Autodesk Inventor part; units mm, degrees
ref_plane "YZ Plane" through (0, 0, 0) normal (1, 0, 0) x (0, 1, 0)
ref_plane "XZ Plane" through (0, 0, 0) normal (0, 1, 0) x (-1, 0, 0)
ref_plane "XY Plane" through (0, 0, 0) normal (0, 0, 1) x (1, 0, 0)
sketch "スケッチ1" plane through (0, 0, 0) normal (0, 1, 0) x (-1, 0, 0)
  arc A0 (-16.7033, 11) -> (16.7033, 11) centre (0, 0) ccw
  line L0 (16.7033, 11) -> (-16.7033, 11)
  point P0 (0, 11)
  dimension "d0" = 40
  dimension "d1" = 11
extrude "押し出し1" add sketch "スケッチ1" along normal blind 6
sketch "スケッチ3" plane through (0, 6, 0) normal (0, 1, 0) x (1, 0, 0)
  arc A0 (2.6833, -3.1) -> (-2.6833, -3.1) centre (0, 0) ccw
  line L0 (-2.6833, -3.1) -> (2.6833, -3.1)
  point P0 (0, -3.1)
  dimension "d12" = 8.2
  dimension "d13" = 3.1
extrude "押し出し2" cut sketch "スケッチ3" against normal blind 6
sketch "スケッチ4" plane through (0, 6, 0) normal (0, 1, 0) x (1, 0, 0)
  circle A0 centre (0, 0) radius 15.5 construction
  line L0 (0, 0) -> (-19.4826, 11.2483) construction
  line L1 (0, 0) -> (29.419, 16.9851) construction
  line L2 (0, 0) -> (0, 25.14) construction
  point P0 (0, 15.5)
  point P1 (-13.4234, 7.75)
  point P2 (-13.4234, 7.75)
  point P3 (0, 15.5)
  point P4 (13.4234, 7.75)
  dimension "d16" = 31
  dimension "d17" = 60
  dimension "d18" = 60
hole "穴2" at (0, 6, -15.5) at (-13.4234, 6, -7.75) at (13.4234, 6, -7.75) direction (0, -1, 0) diameter 3.2 end through all
properties part number "射出_留め具2"
Geometry check sheet. Reference: the model listing, model coordinates, mm. A direction names the side the tool comes from. Give positions to 0.01 mm unless a question says otherwise; leave off trailing zeros. Write each loop counter-clockwise with the first axis right and the second up, starting at its lowest first coordinate (ties: lowest second). Pieces come first, ordered by that corner, then holes. Notation, with made-up numbers: (-13.75, 29) - (17.25, 29) arc R15 cw to (17.25, 43) - close; hole circle Ø6 at (-6.5, 52). An arc over 180 degrees is marked (long way). Use a Markdown table: item, result.
Q1. Section check A-A, the plane x = 0. Enter the section's corners in (y, z).
Computed:
| item | result |
|---|---|
| outline | (0, -20) - (6, -20) - (6, -17.1) - (0, -17.1) - close; (0, -13.9) - (6, -13.9) - (6, -4.1) - (0, -4.1) - close; (0, 3.1) - (6, 3.1) - (6, 11) - (0, 11) - close |
Q2. Draft check along Z on faces 3 (the face through (0.1, 3, -4.1)), 4 (the face through (0, 3, 11)), 5 (the face through (0.3, 6, -4.3)). Enter one of: pulls with the +Z half, pulls with the -Z half, needs draft (parallel to the pull), parting line crosses it, or undercut.
Computed:
| item | result |
|---|---|
| face 3 | undercut |
| face 4 | pulls with the +Z half |
| face 5 | needs draft |
Q3. Thickness scan on L1, parallel to Z at x = 0, y = 4.75; L2, parallel to X at y = 3.8, z = -8; L3, parallel to X at y = 1.25, z = -7.75. Record the ranges inside material, lowest first. Write a range as [from, to].
Computed:
| item | result |
|---|---|
| L1 | z = [-20, -17.1], [-13.9, -4.1], [3.1, 11] |
| L2 | x = [-18.33, -15], [-11.84, 11.84], [15, 18.33] |
| L3 | x = [-18.44, -15.02], [-11.82, 11.82], [15.02, 18.44] |
Q4. Set-up check for faces 1 (the face through (0.3, 0, -4.3)), 2 (the face through (0, 3, 3.1)): record each of +Z, -Z, +X, -X, +Y, -Y from which the full face is reachable in a straight line by a thin tool's end or side.
Computed:
| item | result |
|---|---|
| face 1 | +Z, -Z, +X, -X, -Y |
| face 2 | +Y, -Y |
Q5. Section check D-D, the plane y = 0.85. Enter the section's corners in (x, z), then the cut area to 3 significant figures.
Computed:
| item | result |
|---|---|
| outline | (-16.7, 11) arc R20 ccw (long way) to (16.7, 11) - close; hole circle Ø3.2 at (-13.42, -7.75); hole (-2.68, 3.1) arc R4.1 ccw (long way) to (2.68, 3.1) - close; hole circle Ø3.2 at (0, -15.5); hole circle Ø3.2 at (13.42, -7.75) |
| area | 972 mm² |
Q6. Section check B-B, the plane z = 0. Enter the section's corners in (x, y), then the cut area to 3 significant figures.
Computed:
| item | result |
|---|---|
| outline | (-20, 0) - (-4.1, 0) - (-4.1, 6) - (-20, 6) - close; (4.1, 0) - (20, 0) - (20, 6) - (4.1, 6) - close |
| area | 191 mm² |
Q7. Go/stop test with flat-tipped pins: P1, Ø1.9, axis at x = 0, z = -15.5, coming from the -Y side; P2, Ø1, axis at x = -11, y = 4.5, coming from the -Z side; P3, Ø2, axis at y = 2, z = 4.5, coming from the +X side. Record where each tip stops, or that it passes through.
Computed:
| item | result |
|---|---|
| P1 | passes through |
| P2 | stops at z = -17.02 |
| P3 | stops at x = 19.69 |
Q8. Section check C-C, the plane z = -7.75. Enter the section's corners in (x, y).
Computed:
| item | result |
|---|---|
| outline | (-18.44, 0) - (-15.02, 0) - (-15.02, 6) - (-18.44, 6) - close; (-11.82, 0) - (11.82, 0) - (11.82, 6) - (-11.82, 6) - close; (15.02, 0) - (18.44, 0) - (18.44, 6) - (15.02, 6) - close |
